Could you check a few things on this model? Use its own coordinates, in mm. Face numbers are marked on the shaded views. A direction names the side the tool comes from. Coordinates: 2 decimals unless noted, no trailing zeros. Loops run counter-clockwise (first coordinate to the right, second up) from the corner with the lowest first, then second, coordinate; pieces in that order, holes last. Notation, with made-up numbers: M 67,-27.5 L 84,-27.5 A5 cw 84,-21.5 Z; hole C 49.5,-20 d10. An arc over 180 degrees is marked long. Use one line per item in the form item = value. Start each with the question number.
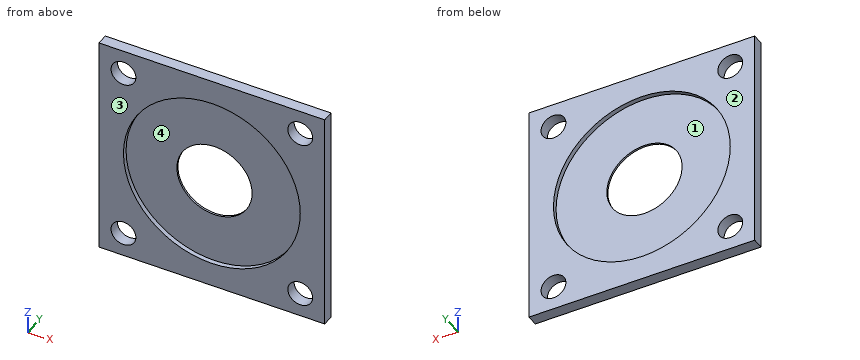
```python
from build123d import *

# Parameters (mm, degrees)
SKETCH2_W           = 60
SKETCH2_H           = 60
SKETCH2_R           = 23.5
SKETCH2_R_2         = 3.3
BOSS_EXTRUDE1_DEPTH = 1.5
BOSS_EXTRUDE2_START = -0.25
SKETCH2_3_R         = 23.5
SKETCH2_3_R_2       = 10
BOSS_EXTRUDE2_DEPTH = 0.5


with BuildPart() as part:
    # Sketch2 → Boss-Extrude1 (new body, symmetric)
    with BuildSketch(Plane(origin=(0, 0, 0), x_dir=(1, 0, 0), z_dir=(0, 1, 0))):
        Rectangle(SKETCH2_W, SKETCH2_H)
        Circle(SKETCH2_R, mode=Mode.SUBTRACT)
        with Locations((23.5, 23.5)):
            Circle(SKETCH2_R_2, mode=Mode.SUBTRACT)
        with Locations((-23.5, 23.5)):
            Circle(SKETCH2_R_2, mode=Mode.SUBTRACT)
        with Locations((23.5, -23.5)):
            Circle(SKETCH2_R_2, mode=Mode.SUBTRACT)
        with Locations((-23.5, -23.5)):
            Circle(SKETCH2_R_2, mode=Mode.SUBTRACT)
    extrude(amount=BOSS_EXTRUDE1_DEPTH, both=True)

    # Sketch2_3 → Boss-Extrude2 (add)
    with BuildSketch(Plane(origin=(0, 0, 0), x_dir=(1, 0, 0), z_dir=(0, 1, 0)).offset(BOSS_EXTRUDE2_START)):
        Circle(SKETCH2_3_R)
        Circle(SKETCH2_3_R_2, mode=Mode.SUBTRACT)
    extrude(amount=BOSS_EXTRUDE2_DEPTH)


solid = part.part
```
Item 1: I want a section at B-B (z = 0). Write out the boundary of the cut face in (x, y).
Item 2: For the marked faces 1 and 2, which set-ups out of +Z, -Z, +X, -X, +Y, -Y let a thin tool reach every point of the face, with its end or its side?
Item 3: I want a section at D-D (x = 18). Write out the boundary of the cut face in (y, z), plus the area to 3 significant figures.
Item 4: Please list where these lines run through material, in increasing order: line 1 along Z through (x, y) = (25.5, -0.1); line 2 along X through (y, z) = (0.05, 0).
Item 5: I'm going to push flat-ended pins straight in: P1, Ø10, axis at x = 8, z = 12, coming from the +Y side; P2, Ø1.5, axis at x = -21.5, z = 22.5, coming from the -Y side. Where does each tip first touch, or does it pass through?
Item 6: I want a section at A-A (x = 0). Write out the boundary of the cut face in (y, z).
Item 7: Thinking about a two-plate mould opening in X: for the marked faces 3 and 4, which applies, pulls with the +X half, pulls with the -X half, needs draft (parallel to the pull), parting line crosses it, or undercut?
Item 8: I want a section at C-C (z = -17). Write out the boundary of the cut face in (x, y), plus the area to 3 significant figures.
Worked answers:
q1.outline = M -30,-1.5 L -23.5,-1.5 L -23.5,-0.25 L -10,-0.25 L -10,0.25 L -23.5,0.25 L -23.5,1.5 L -30,1.5 Z; M 10,-0.25 L 23.5,-0.25 L 23.5,-1.5 L 30,-1.5 L 30,1.5 L 23.5,1.5 L 23.5,0.25 L 10,0.25 Z
q2.face_1 = +Y
q2.face_2 = +Z, -Z, +X, -X, +Y
q3.outline = M -1.5,-30 L 1.5,-30 L 1.5,-15.11 L 0.25,-15.11 L 0.25,15.11 L 1.5,15.11 L 1.5,30 L -1.5,30 L -1.5,15.11 L -0.25,15.11 L -0.25,-15.11 L -1.5,-15.11 Z
q3.area = 104 mm²
q4.line_1 = -30 to -26.12, -20.88 to 20.88, 26.12 to 30
q4.line_2 = -30 to -10, 10 to 30
q5.P1 = 0.25
q5.P2 = through
q6.outline = M -1.5,-30 L 1.5,-30 L 1.5,-23.5 L 0.25,-23.5 L 0.25,-10 L -0.25,-10 L -0.25,-23.5 L -1.5,-23.5 Z; M -1.5,23.5 L -0.25,23.5 L -0.25,10 L 0.25,10 L 0.25,23.5 L 1.5,23.5 L 1.5,30 L -1.5,30 Z
q7.face_3 = needs draft
q7.face_4 = undercut
q8.outline = M -30,-1.5 L -16.22,-1.5 L -16.22,-0.25 L 16.22,-0.25 L 16.22,-1.5 L 30,-1.5 L 30,1.5 L 16.22,1.5 L 16.22,0.25 L -16.22,0.25 L -16.22,1.5 L -30,1.5 Z
q8.area = 98.9 mm²
